```python
from build123d import *

# Parameters (mm, degrees)
ESQUISSE1_R        = 2.75
BOSS_EXTRU_1_DEPTH = 30
ESQUISSE2_W        = 5.5
ESQUISSE2_H        = 5.5
BOSS_EXTRU_2_DEPTH = 5
ESQUISSE3_R        = 7.5
BOSS_EXTRU_3_DEPTH = 0.5
D_ME1_FACE_RADIUS  = 7.5
D_ME1_HEIGHT       = 2.5


with BuildPart() as part:
    # Esquisse1 → Boss.-Extru.1 (new body)
    with BuildSketch(Plane.XY):
        Circle(ESQUISSE1_R)
    extrude(amount=BOSS_EXTRU_1_DEPTH)

    # Esquisse2 → Boss.-Extru.2 (add)
    with BuildSketch(Plane(origin=(0, 0, 0), x_dir=(-1, 0, 0), z_dir=(0, 0, -1))):
        Rectangle(ESQUISSE2_W, ESQUISSE2_H)
    extrude(amount=BOSS_EXTRU_2_DEPTH)

    # Esquisse3 → Boss.-Extru.3 (add)
    with BuildSketch(Plane(origin=(0, 0, -5), x_dir=(-1, 0, 0), z_dir=(0, 0, -1))):
        Circle(ESQUISSE3_R)
    extrude(amount=BOSS_EXTRU_3_DEPTH)

    # Dôme1: a dome of height H over a round flat face of radius A is a cap of a sphere of radius (A * A + H * H) / (2 * H)
    d_me1_r = (D_ME1_FACE_RADIUS * D_ME1_FACE_RADIUS + D_ME1_HEIGHT * D_ME1_HEIGHT) / (2 * D_ME1_HEIGHT)
    d_me1_base = Plane((0, 0, -5.5), z_dir=(0, 0, -1))
    with Locations(d_me1_base.offset(D_ME1_HEIGHT - d_me1_r)):
        d_me1_ball = Sphere(d_me1_r, mode=Mode.PRIVATE)
    add(split(d_me1_ball, bisect_by=d_me1_base, keep=Keep.TOP, mode=Mode.PRIVATE))


solid = part.part
```
Geometry check sheet. Reference: the model listing, model coordinates, mm. A direction names the side the tool comes from. Coordinates: 2 decimals unless noted, no trailing zeros. Loops run counter-clockwise (first coordinate to the right, second up) from the corner with the lowest first, then second, coordinate; pieces in that order, holes last.
Item 1: Sectioned sample at A-A, the plane x = -1.25. Record the boundary of the cut face in (y, z).
Item 2: Sectioned sample at B-B, the plane z = 11.5. Record the boundary of the cut face in (x, y), then the cut area to 3 significant figures.
Item 3: Sectioned sample at D-D, the plane y = 5. Record the boundary of the cut face in (x, z).
Item 4: Sectioned sample at C-C, the plane y = -5.5. Record the boundary of the cut face in (x, z).
Item 5: Access from +Z, -Z, +X, -X, +Y, -Y to the whole of each face (thin tool, end or side, straight path). Record for faces 1 (the face through (2.75, 0, -2)), 2 (the face through (2.2, -2.1, 0)), 3 (the face through (-2.75, 0, -2)).
Item 6: Go/stop test with flat-tipped pins: pin 1 Ø5.5 at (x, z) = (1, -2) entering from +Y; pin 2 Ø4 at (x, z) = (-1, -1.5) entering from -Y; pin 3 Ø5 at (x, z) = (4.5, 16) entering from +Y; pin 4 Ø4 at (y, z) = (-1, -3.5) entering from +X. Record where each tip stops, or that it passes through.
Item 7: Thickness scan on line 1 (Z direction, x = -0.25, y = -6.25); line 2 (Y direction, x = 0.5, z = 18); line 3 (X direction, y = 2, z = 13). Record the ranges inside material, lowest first.
Check result:
1. outline: (-7.4, -5.5) arc R12.44 ccw to (7.4, -5.5) - (7.4, -5) - (2.75, -5) - (2.75, 0) - (2.45, 0) - (2.45, 30) - (-2.45, 30) - (-2.45, 0) - (-2.75, 0) - (-2.75, -5) - (-7.4, -5) - close
2. outline: circle Ø5.5 at (0, 0)
2. area: 23.8 mm2
3. outline: (-5.59, -5.5) arc R11.46 ccw to (5.59, -5.5) - (5.59, -5) - (-5.59, -5) - close
4. outline: (-5.1, -5.5) arc R11.22 ccw to (5.1, -5.5) - (5.1, -5) - (-5.1, -5) - close
5. face 1: +Z, +X, +Y, -Y
5. face 2: +Z, +X, -Y
5. face 3: +Z, -X, +Y, -Y
6. pin 1: stops at y = 2.75
6. pin 2: stops at y = -2.75
6. pin 3: stops at y = 1.89
6. pin 4: stops at x = 7.5
7. line 1: z = -6.32 to -5
7. line 2: y = -2.7 to 2.7
7. line 3: x = -1.89 to 1.89
